Work out the finished part from the listing and answer in its coordinate system (mm). A direction names the side the tool comes from. Round coordinates to 2 decimals unless told otherwise and drop trailing zeros. Order: outer loops, then holes, each group sorted by start corner. A loop starts at its lowest first (then second) coordinate and runs counter-clockwise, first axis right, second up. Notation, with made-up numbers: M -36.5,20 L 2.5,20 A18 cw 2.5,31 Z; hole C 19.5,5.5 d1. An arc over 180 degrees is marked long. Answer as a JSON object with one key per item and string values. Group by question number.
from build123d import *

# Parameters (mm, degrees)
CHAMFER1_SIZE  = 0.5
CHAMFER1_SIZE2 = 0.866025404


with BuildPart() as part:
    # Sketch2 → Revolve1 (revolve)
    with BuildSketch(Plane(origin=(0, 0, 0), x_dir=(0, 0, -1), z_dir=(1, 0, 0))):
        Polygon((27, 0), (27, 1.1), (28.5, 1.1), (28.5, 3.1), (27, 3.1), (27, 4.5), (25, 4.5), (25, -1.5), (28.5, -1.5), (28.5, -1.1), (27, -1.1), align=None)
    revolve(axis=Axis((0, 0, 0), (0, 1, 0)))

    # Chamfer1
    chamfer1_edges = [part.edges().sort_by_distance(p)[0] for p in [
        (0, 4.5, 25),
    ]]
    chamfer1_side = [part.faces().sort_by_distance(p)[0] for p in [
        (0, 4.5, 26.236324676),
    ]]
    chamfer(chamfer1_edges, length=CHAMFER1_SIZE, length2=CHAMFER1_SIZE2, reference=chamfer1_side[0])


solid = part.part
Item 1: Find section C-C (y = 2.4). Give the vertices of the cut face in (x, z), and give its area (3 significant figures).
Item 2: Find section B-B (z = 0). Give the vertices of the cut face in (x, y).
Item 3: Each of these flat-tipped pins is pushed along its axis until it touches: pin 1 (2 mm diameter, centred on y = 2.5, z = -17, fed in from -X); pin 2 (1 mm diameter, centred on y = 1.5, z = 4, fed in from +X); pin 3 (3 mm diameter, centred on x = 3.5, y = 0, fed in from +Z). Where does it stop, or does it pass through?
Item 4: The mould has two halves that part along Z. Classify faces 1 (the cylindrical face through (26.36, 0.02, 5.85)), 2 (the cylindrical face through (-7.509, 1.031, -23.846)), 3 (the flat face through (25.2, -1.5, -0.1)): +Z half, -Z half, draft (parallel to the pull), parting line (faces both ways), or undercut.
Item 5: Find section A-A (x = 0). Give the vertices of the cut face in (y, z), and give its area (3 significant figures).
Item 6: A tool of negligible diameter and unlimited length cuts with its end or side. For faces 4 (the cylindrical face through (26.36, 3.81, 5.85)), 5 (the cylindrical face through (10.916, 2.114, -26.327)), 6 (the flat face through (10.4, 1.1, 25.2)), from which of +Z, -Z, +X, -X, +Y, -Y can it reach the whole face along a straight path? Write none if from no direction.
Item 7: Consider L1, parallel to Z at x = 0, y = 2.4; L2, parallel to X at y = -0.5, z = 0.5 (3 decimals); L3, parallel to Z at x = 0, y = 0.45. Determine where each line is inside the solid, lowest interval first.
Responses:
{
 "1": {"outline": "C 0,0 d57; hole C 0,0 d50", "area": "588 mm^2"},
 "2": {"outline": "M -28.5,-1.5 L -25,-1.5 L -25,3.63 L -25.5,4.5 L -27,4.5 L -27,3.1 L -28.5,3.1 L -28.5,1.1 L -27,1.1 L -27,-1.1 L -28.5,-1.1 Z; M 25,-1.5 L 28.5,-1.5 L 28.5,-1.1 L 27,-1.1 L 27,1.1 L 28.5,1.1 L 28.5,3.1 L 27,3.1 L 27,4.5 L 25.5,4.5 L 25,3.63 Z"},
 "3": {"pin 1": "stops at x = -23.58", "pin 2": "stops at x = 28.28", "pin 3": "stops at z = 28.39"},
 "4": {"face 1": "parting line", "face 2": "undercut", "face 3": "draft"},
 "5": {"outline": "M -1.5,-28.5 L -1.1,-28.5 L -1.1,-27 L 1.1,-27 L 1.1,-28.5 L 3.1,-28.5 L 3.1,-27 L 4.5,-27 L 4.5,-25.5 L 3.63,-25 L -1.5,-25 Z; M -1.5,25 L 3.63,25 L 4.5,25.5 L 4.5,27 L 3.1,27 L 3.1,28.5 L 1.1,28.5 L 1.1,27 L -1.1,27 L -1.1,28.5 L -1.5,28.5 Z", "area": "30.8 mm^2"},
 "6": {"face 4": "+Y", "face 5": "+Y, -Y", "face 6": "none"},
 "7": {"L1": "z = -28.5 to -25, 25 to 28.5", "L2": "x = -26.995 to -24.995, 24.995 to 26.995", "L3": "z = -27 to -25, 25 to 27"}
}
